Autodesk Inventor part; units mm, degrees
ref_plane "YZ Plane" through (0, 0, 0) normal (1, 0, 0) x (0, 1, 0)
ref_plane "XZ Plane" through (0, 0, 0) normal (0, 1, 0) x (-1, 0, 0)
ref_plane "XY Plane" through (0, 0, 0) normal (0, 0, 1) x (1, 0, 0)
sketch "Boceto1" plane through (0, 0, 0) normal (0, 1, 0) x (-1, 0, 0)
  circle A0 centre (0, 0) radius 5.65
  circle A1 centre (0, 0) radius 8.65
  line L0 (0, 0) -> (6.6609, -5.5186)
  line L1 (0, 0) -> (5.5186, 6.6609)
  line L2 (3.6046, 4.3508) -> (7.4762, 4.3508)
  line L3 (4.3508, -3.6046) -> (7.8632, -3.6046)
  point P0 (-0.8522, 8.6079)
  point P1 (-0.8522, -8.6079)
  point P2 (3.6046, 4.3508)
  point P3 (4.3508, -3.6046)
  dimension "d0" = 11.3
  dimension "d1" = 3
  dimension "d5" = 90
extrude "Extrusión1" add sketch "Boceto1" along normal blind 3 contours A0 L0 A1 L1 | L1 A1 L2 | L3 A1 L0
properties part number "Rubberfoot" material "Caucho, Silicona"
For this review, take the finished solid that the model builds, in its own axes (mm). A direction names the side the tool comes from. Give positions to 0.01 mm unless a question says otherwise; leave off trailing zeros. Order: outer loops, then holes, each group sorted by start corner. A loop starts at its lowest first (then second) coordinate and runs counter-clockwise, first axis right, second up. Notation, with made-up numbers: M 70,-7 L 79,-7 A25 ccw 79,17 Z; hole C -18.5,-36 d11. An arc over 180 degrees is marked long. Answer in a Markdown table with one row per item. Add a question column.
(1) Consider section B-B on z = -5. State the section outline as (x, y) points, and give its area (3 significant figures).
(2) Consider section A-A on x = 0. State the section outline as (y, z) points.
(3) For pin 1 (4 mm diameter, centred on x = -1, z = 4, fed in from -Y); pin 2 (1 mm diameter, centred on x = 3, y = 1.5, fed in from -Z); pin 3 (1.5 mm diameter, centred on x = -5.5, y = 1, fed in from +Z), all flat-tipped, find the tip position at first contact; note any pin that passes through.
(4) Wall thickness on probe 1 along Z at (x, y) = (0, 1.8); probe 2 along X at (y, z) = (1.6, 0); probe 3 along Z at (x, y) = (-4, 2.5): over which ranges is each line inside the solid? List them lowest first. Write a range as [from, to].
(5) For faces 1 (the face through (-6, 1, 4.351)), 2 (the face through (5.605, 1.479, -0.713)), list the 3-axis set-ups (+Z, -Z, +X, -X, +Y, -Y) from which the entire face can be reached by the end or side of a thin tool; tool diameter is ignored.
(6) Consider section C-C on z = 0. State the section outline as (x, y) points, and give its area (3 significant figures).
(7) Consider section D-D on x = 6. State the section outline as (y, z) points, and give its area (3 significant figures).
Evaluation:
| question | item | result |
|---|---|---|
| 1 | outline | M -7.06,0 L -2.63,0 L -2.63,3 L -7.06,3 Z; M 2.63,0 L 7.06,0 L 7.06,3 L 2.63,3 Z |
| 1 | area | 26.6 mm^2 |
| 2 | outline | M 0,-8.65 L 3,-8.65 L 3,-5.65 L 0,-5.65 Z; M 0,5.65 L 3,5.65 L 3,8.65 L 0,8.65 Z |
| 3 | pin 1 | stops at y = 0 |
| 3 | pin 2 | stops at z = -8.28 |
| 3 | pin 3 | stops at z = 7.23 |
| 4 | probe 1 | z = [-8.65, -5.65], [5.65, 8.65] |
| 4 | probe 2 | x = [5.65, 8.65] |
| 4 | probe 3 | z = [-7.67, -3.99], [4.35, 7.67] |
| 5 | face 1 | -X, +Y, -Y |
| 5 | face 2 | +Y, -Y |
| 6 | outline | M 5.65,0 L 8.65,0 L 8.65,3 L 5.65,3 Z |
| 6 | area | 9.00 mm^2 |
| 7 | outline | M 0,-6.23 L 3,-6.23 L 3,6.23 L 0,6.23 Z |
| 7 | area | 37.4 mm^2 |
